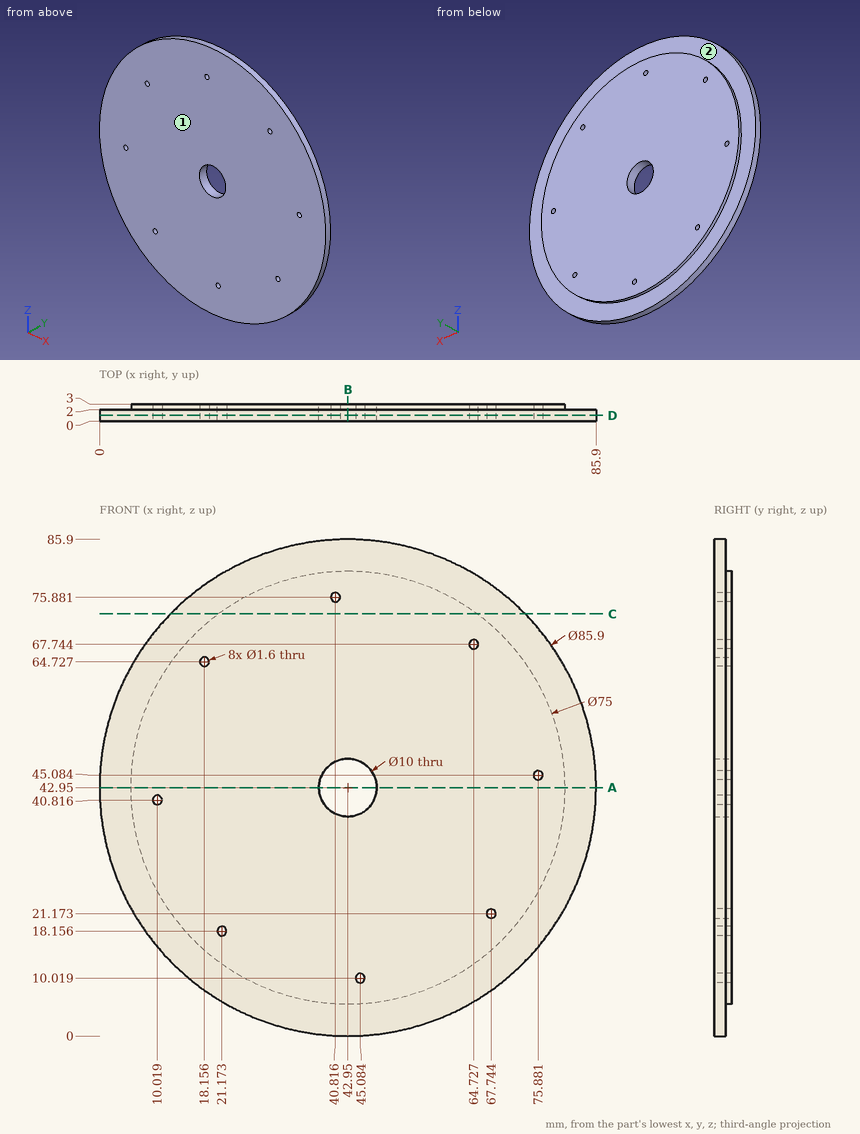
Geometry: see drawing. Coordinates: mm, zero at the bounding-box minimum. A direction names the side the tool comes from. Round coordinates to 2 decimals unless told otherwise and drop trailing zeros. Order: outer loops, then holes, each group sorted by start corner. A loop starts at its lowest first (then second) coordinate and runs counter-clockwise, first axis right, second up. Notation, with made-up numbers: (47, -13.75) -> (92, -13.75) arc R26 ccw to (92, 9.25) -> close; hole circle Ø5 at (-38.5, 6). An arc over 180 degrees is marked (long way). Answer as CSV lines item,"result".
Item 1: Reachability of the marked faces 1 and 2 from +Z, -Z, +X, -X, +Y, -Y: full face, straight path, thin tool, end or side. Return the list, or none.
A:
face 1,"+Z, -Z, +X, -X, -Y"
face 2,"+Y"
Item 2: Section C-C, the plane z = 73. Return loops of the section in (x, y).
A:
outline,"(12.26, 0) -> (73.64, 0) -> (73.64, 2) -> (65.38, 2) -> (65.38, 3) -> (20.52, 3) -> (20.52, 2) -> (12.26, 2) -> close"
Item 3: Section D-D, the plane y = 1.05. Count the separate pieces of the cut face and the enclosed holes in it, plus the area to 3 significant figures.
A:
separate pieces,"1"
enclosed holes,"9"
area,"5,700 mm²"
Item 4: Pin query (flat end, axial travel): pin 1 Ø1.8 at (x, z) = (67.74, 21.17) entering from -Y; pin 2 Ø9 at (x, z) = (42.95, 42.95) entering from -Y. Return the tip coordinate at first contact, or that it passes through.
A:
pin 1,"y = 0"
pin 2,"through"
Item 5: Line query: L1, parallel to Z at x = 68, y = 2.2 (1 decimal); L2, parallel to Z at x = 47, y = 2.25 (1 decimal); L3, parallel to Y at x = 4, z = 54.5. Output: solid intervals per line, ascending.
A:
L1,"15 to 20.4, 21.9 to 70.9"
L2,"5.7 to 40, 45.9 to 80.2"
L3,"0 to 2"
Item 6: Section A-A, the plane z = 42.95. Return loops of the section in (x, y).
A:
outline,"(0, 0) -> (37.95, 0) -> (37.95, 3) -> (5.45, 3) -> (5.45, 2) -> (0, 2) -> close; (47.95, 0) -> (85.9, 0) -> (85.9, 2) -> (80.45, 2) -> (80.45, 3) -> (47.95, 3) -> close"
Item 7: Section B-B, the plane x = 42.95. Return loops of the section in (y, z), plus the area to 3 significant figures.
A:
outline,"(0, 0) -> (2, 0) -> (2, 5.45) -> (3, 5.45) -> (3, 37.95) -> (0, 37.95) -> close; (0, 47.95) -> (3, 47.95) -> (3, 80.45) -> (2, 80.45) -> (2, 85.9) -> (0, 85.9) -> close"
area,"217 mm²"
